Could you check a few things on this model? Use its own coordinates, in mm. A direction names the side the tool comes from. Round coordinates to 2 decimals unless told otherwise and drop trailing zeros. Return JSON: item names as keys, results as strings.
from build123d import *

# Parameters (mm, degrees)
F0_R     = 3.362501
F1_DEPTH = 165.1


with BuildPart() as f1:
    # F0 (on Top) → F1 (new body, symmetric)
    with BuildSketch(Plane.XY):
        with BuildLine():
            ThreePointArc((-7.291522, 15.377258), (-8.527575, 14.551354), (-9.985599, 14.261335))
            Line((-9.985599, 14.261335), (-12.900292, 14.261335))
            ThreePointArc((-12.900292, 14.261335), (-14.358316, 14.551354), (-15.594369, 15.377258))
            Line((-15.594369, 15.377258), (-17.43985, 17.222739))
            ThreePointArc((-17.43985, 17.222739), (-17.852803, 19.29879), (-16.092812, 20.474778))
            Line((-16.092812, 20.474778), (-14.358316, 20.474778))
            Line((-14.358316, 20.474778), (-14.325965, 20.474778))
            ThreePointArc((-14.325965, 20.474778), (-13.56835, 21.248399), (-14.325965, 22.02202))
            Line((-14.325965, 22.02202), (-14.358316, 22.02202))
            Line((-14.358316, 22.02202), (-14.996286, 22.02202))
            ThreePointArc((-14.996286, 22.02202), (-15.544549, 21.480792), (-16.092812, 22.02202))
            Line((-16.092812, 22.02202), (-19.230427, 22.02202))
            ThreePointArc((-19.230427, 22.02202), (-19.781686, 21.470761), (-20.332945, 22.02202))
            ThreePointArc((-20.332945, 22.02202), (-23.027022, 20.906097), (-24.142945, 18.21202))
            Line((-24.142945, 18.21202), (-24.142945, 17.126744))
            Line((-24.142945, 17.126744), (-24.142945, 13.971887))
            ThreePointArc((-24.142945, 13.971887), (-23.587106, 13.424695), (-24.142945, 12.877503))
            Line((-24.142945, 12.877503), (-24.142945, 12.23739))
            ThreePointArc((-24.142945, 12.23739), (-23.369324, 11.481574), (-22.595703, 12.23739))
            Line((-22.595703, 12.23739), (-22.595703, 13.971887))
            ThreePointArc((-22.595703, 13.971887), (-21.419715, 15.731877), (-19.343665, 15.318925))
            Line((-19.343665, 15.318925), (-18.091092, 14.066352))
            ThreePointArc((-18.091092, 14.066352), (-17.265188, 12.830299), (-16.975169, 11.372275))
            Line((-16.975169, 11.372275), (-16.975169, 5.601584))
            ThreePointArc((-16.975169, 5.601584), (-19.785436, 2.791317), (-22.595703, 5.601584))
            Line((-22.595703, 5.601584), (-22.595703, 6.406649))
            ThreePointArc((-22.595703, 6.406649), (-23.369324, 7.18027), (-24.142945, 6.406649))
            Line((-24.142945, 6.406649), (-24.142945, 5.771259))
            Line((-24.142945, 5.771259), (-24.142945, 1.526558))
            ThreePointArc((-24.142945, 1.526558), (-23.589161, 0.979289), (-24.142945, 0.43202))
            ThreePointArc((-24.142945, 0.43202), (-23.027022, -2.262057), (-20.332945, -3.37798))
            ThreePointArc((-20.332945, -3.37798), (-19.783762, -2.823095), (-19.234579, -3.37798))
            Line((-19.234579, -3.37798), (-15.451114, -3.37798))
            ThreePointArc((-15.451114, -3.37798), (-14.904715, -2.837846), (-14.358316, -3.37798))
            ThreePointArc((-14.358316, -3.37798), (-13.597129, -2.60328), (-14.358316, -1.82858))
            Line((-14.358316, -1.82858), (-16.090654, -1.82858))
            ThreePointArc((-16.090654, -1.82858), (-17.850645, -0.652592), (-17.437693, 1.423458))
            Line((-17.437693, 1.423458), (-15.594369, 3.266782))
            ThreePointArc((-15.594369, 3.266782), (-14.358316, 4.092686), (-12.900292, 4.382705))
            Line((-12.900292, 4.382705), (-9.985599, 4.382705))
            ThreePointArc((-9.985599, 4.382705), (-8.527575, 4.092686), (-7.291522, 3.266782))
            Line((-7.291522, 3.266782), (-5.448198, 1.423458))
            ThreePointArc((-5.448198, 1.423458), (-5.035246, -0.652592), (-6.795236, -1.82858))
            Line((-6.795236, -1.82858), (-8.527575, -1.82858))
            ThreePointArc((-8.527575, -1.82858), (-9.144781, -2.60328), (-8.527575, -3.37798))
            Line((-8.527575, -3.37798), (-7.895813, -3.37798))
            ThreePointArc((-7.895813, -3.37798), (-7.345525, -2.832718), (-6.795236, -3.37798))
            Line((-6.795236, -3.37798), (-3.641811, -3.37798))
            ThreePointArc((-3.641811, -3.37798), (-3.097378, -2.833547), (-2.552945, -3.37798))
            ThreePointArc((-2.552945, -3.37798), (0.141132, -2.262057), (1.257055, 0.43202))
            ThreePointArc((1.257055, 0.43202), (0.717674, 0.97812), (1.257055, 1.52422))
            Line((1.257055, 1.52422), (1.257055, 4.674311))
            ThreePointArc((1.257055, 4.674311), (0.713538, 5.22368), (1.257055, 5.773049))
            Line((1.257055, 5.773049), (1.257055, 6.406649))
            ThreePointArc((1.257055, 6.406649), (0.482355, 7.126711), (-0.292345, 6.406649))
            Line((-0.292345, 6.406649), (-0.292345, 4.674311))
            ThreePointArc((-0.292345, 4.674311), (-1.468333, 2.91432), (-3.544384, 3.327273))
            Line((-3.544384, 3.327273), (-5.387707, 5.170596))
            ThreePointArc((-5.387707, 5.170596), (-6.213612, 6.406649), (-6.503631, 7.864673))
            Line((-6.503631, 7.864673), (-6.503631, 10.779367))
            ThreePointArc((-6.503631, 10.779367), (-6.213612, 12.23739), (-5.387707, 13.473443))
            Line((-5.387707, 13.473443), (-3.544384, 15.316767))
            ThreePointArc((-3.544384, 15.316767), (-1.468333, 15.729719), (-0.292345, 13.969729))
            Line((-0.292345, 13.969729), (-0.292345, 12.23739))
            ThreePointArc((-0.292345, 12.23739), (0.482355, 11.501425), (1.257055, 12.23739))
            Line((1.257055, 12.23739), (1.257055, 12.877529))
            ThreePointArc((1.257055, 12.877529), (0.710955, 13.423629), (1.257055, 13.969729))
            Line((1.257055, 13.969729), (1.257055, 17.117185))
            ThreePointArc((1.257055, 17.117185), (0.705999, 17.664602), (1.257055, 18.21202))
            ThreePointArc((1.257055, 18.21202), (0.141132, 20.906097), (-2.552945, 22.02202))
            ThreePointArc((-2.552945, 22.02202), (-3.108248, 21.525639), (-3.663551, 22.02202))
            Line((-3.663551, 22.02202), (-6.793078, 22.02202))
            ThreePointArc((-6.793078, 22.02202), (-7.33931, 21.481453), (-7.885542, 22.02202))
            Line((-7.885542, 22.02202), (-8.527575, 22.02202))
            Line((-8.527575, 22.02202), (-8.599148, 22.02202))
            ThreePointArc((-8.599148, 22.02202), (-9.33781, 21.248399), (-8.599148, 20.474778))
            Line((-8.599148, 20.474778), (-8.527575, 20.474778))
            Line((-8.527575, 20.474778), (-6.793078, 20.474778))
            ThreePointArc((-6.793078, 20.474778), (-5.033088, 19.29879), (-5.44604, 17.222739))
            Line((-5.44604, 17.222739), (-7.291522, 15.377258))
        make_face()
        with Locations((-11.442945, 9.32202)):
            Circle(F0_R, mode=Mode.SUBTRACT)
        with BuildLine():
            ThreePointArc((-8.599148, 20.474778), (-8.563361, 20.473951), (-8.527575, 20.474778))
            Line((-8.527575, 20.474778), (-8.599148, 20.474778))
        make_face()
        with BuildLine():
            Line((-14.325965, 20.474778), (-14.358316, 20.474778))
            ThreePointArc((-14.358316, 20.474778), (-14.34214, 20.474609), (-14.325965, 20.474778))
        make_face()
        with BuildLine():
            ThreePointArc((-8.527575, 22.02202), (-8.563361, 22.022847), (-8.599148, 22.02202))
            Line((-8.599148, 22.02202), (-8.527575, 22.02202))
        make_face()
        with BuildLine():
            Line((-14.358316, 22.02202), (-14.325965, 22.02202))
            ThreePointArc((-14.325965, 22.02202), (-14.34214, 22.022189), (-14.358316, 22.02202))
        make_face()
    extrude(amount=F1_DEPTH, both=True)


solid = f1.part
1) Will these pins go through, and if not, where does the flat tip stop? pin 1 Ø0.9 at (x, z) = (-11.5, -57) entering from +Y; pin 2 Ø2.5 at (y, z) = (9.5, -66) entering from +X; pin 3 Ø3 at (y, z) = (8, -58) entering from -X.
Return value:
{"pin 1": "y = 14.26", "pin 2": "x = -6.5", "pin 3": "x = -24.14"}
2) Thinking about a two-plate mould opening in X: for faces 3 (the face through (-13.921, 11.595, -2.311)), 4 (the face through (-16.975, 9, 2)), 5 (the face through (-14, 12, -165.1)), which applies, pulls with the +X half, pulls with the -X half, needs draft (parallel to the pull), parting line crosses it, or undercut?
Return value:
{"face 3": "undercut", "face 4": "undercut", "face 5": "needs draft"}
3) For faces 1 (the face through (-14, 12, 165.1)), 2 (the face through (-19.724, 2.792, 2.311)), which set-ups out of +Z, -Z, +X, -X, +Y, -Y let a thin tool reach every point of the face, with its end or its side?
Return value:
{"face 1": "+Z, +X, -X, +Y, -Y", "face 2": "+Z, -Z"}
4) If I drill on probe 1 along Y at (x, z) = (-6.75, 79); probe 2 along X at (y, z) = (3.75, -138); probe 3 along Y at (x, z) = (-11.5, -30), over which ranges is the centre line in solid material (lowest first)? Write a range as [from, to].
Return value:
{"probe 1": "[-3.38, -1.83], [2.73, 15.92], [20.47, 22.02]", "probe 2": "[-24.14, -21.9], [-17.67, -15], [-7.88, -3.97], [-0.53, 1.26]", "probe 3": "[4.38, 5.96], [12.68, 14.26]"}
